Autodesk Inventor part; units mm, degrees
ref_plane "YZ Plane" through (0, 0, 0) normal (1, 0, 0) x (0, 1, 0)
ref_plane "XZ Plane" through (0, 0, 0) normal (0, 1, 0) x (-1, 0, 0)
ref_plane "XY Plane" through (0, 0, 0) normal (0, 0, 1) x (1, 0, 0)
sketch "スケッチ1" plane through (0, 0, 0) normal (0, 0, 1) x (1, 0, 0)
  circle A0 centre (0, 0) radius 18.4
extrude "押し出し1" add sketch "スケッチ1" along normal blind 24
sketch "スケッチ2" plane through (0, 0, 0) normal (0, 0, -1) x (-1, 0, 0)
  circle A0 centre (0, 0) radius 17.4
  dimension "d3" = 34.8
extrude "押し出し2" add sketch "スケッチ2" along normal blind 30.7
sketch "スケッチ3" plane through (0, 0, -30.7) normal (0, 0, -1) x (-1, 0, 0)
  circle A0 centre (0, 0) radius 17
  dimension "d6" = 34
extrude "押し出し3" add sketch "スケッチ3" along normal blind 15.4
sketch "スケッチ4" plane through (0, 0, 24) normal (0, 0, 1) x (1, 0, 0)
  circle A0 centre (0, -7) radius 6
  circle A1 centre (0, -7) radius 3
  point P0 (0, 0)
  point P1 (-15.5, 0)
  point P2 (0, 0)
  point P3 (-7.75, -13.4234)
  point P4 (7.75, -13.4234)
  point P5 (15.5, 0)
  point P6 (7.75, 13.4234)
  point P7 (-7.75, 13.4234)
  dimension "d11" = 360
  dimension "d13" = 15.5
  dimension "d14" = 7
  dimension "d15" = 12
  dimension "d16" = 6
extrude "押し出し4" add sketch "スケッチ4" along normal blind 6
extrude "押し出し5" add sketch "スケッチ4" along normal blind 22 contours A1
sketch "スケッチ5" plane through (0, -7, 46) normal (0, 0, 1) x (1, 0, 0)
  circle A0 centre (0, 0) radius 3
  line L0 (0, 2.4) -> (1.8, 2.4)
  line L1 (0, 2.4) -> (-1.8, 2.4)
  point P0 (0, 7)
  dimension "d21" = 6
  dimension "d22" = 2.4
extrude "押し出し6" cut sketch "スケッチ5" against normal blind 12 contours L0 L1 A0 picked at (-1.016, 2.5094)
sketch "スケッチ6" plane through (0, 0, 24) normal (0, 0, 1) x (1, 0, 0)
  point P0 (0, 0)
  point P1 (-15.5, 0)
  point P2 (-7.75, -13.4234)
  point P3 (7.75, -13.4234)
  point P4 (15.5, 0)
  point P5 (7.75, 13.4234)
  point P6 (-7.75, 13.4234)
  dimension "d25" = 15.5
  dimension "d28" = 360
hole "穴1" at (7.75, 13.4234, 24) at (-7.75, 13.4234, 24) at (-15.5, 0, 24) at (-7.75, -13.4234, 24) at (7.75, -13.4234, 24) at (15.5, 0, 24) direction (0, 0, -1) diameter 2.459 depth 8.8 tip angle 118
properties part number "Metal Gearmotor"
Read the model definition and answer for the solid it produces. Units are mm, in the model's axes. A direction names the side the tool comes from. Give positions to 0.01 mm unless a question says otherwise; leave off trailing zeros. Order: outer loops, then holes, each group sorted by start corner. A loop starts at its lowest first (then second) coordinate and runs counter-clockwise, first axis right, second up. Notation, with made-up numbers: (82.5, -28.5) -> (126.5, -28.5) arc R31 ccw to (126.5, -4.5) -> close; hole circle Ø8 at (41.5, 5.25). An arc over 180 degrees is marked (long way). One line per item, written item: value. Start each with the question number.
(1) The part is cut by section D-D (z = -17). Determine the outline of the cut face in (x, y).
(2) The part is cut by section C-C (y = -3). Determine the outline of the cut face in (x, z).
(3) A tool of negligible diameter and unlimited length cuts with its end or side. For faces 1 (the flat face through (0, -4.6, 40)), 2 (the cylindrical face through (-14.6, 11.2, 11.8)), 3 (the flat face through (0, 0, -46.1)), 4 (the cylindrical face through (8.5, 14.4, 19.5)), 5 (the flat face through (14, 11, 0)), from which of +Z, -Z, +X, -X, +Y, -Y can it reach the whole face along a straight path? Write none if from no direction.
(4) For a pull along X with two mould halves and no side action, classify faces 6 (the cylindrical face through (-6.55, 13.69, 19.54)), 7 (the cylindrical face through (-9.139, -14.334, -38.292)), 8 (the flat face through (-15.4, -7.7, -30.7)), 9 (the cylindrical face through (8.5, -12.45, 19.54)) as released by +X, released by -X, zero draft, split by the parting line, or undercut.
(5) The part is cut by section A-A (x = 0). Determine the outline of the cut face in (y, z), and give its area (3 significant figures).
(6) Flat-ended cylindrical pins translate along their axes: P1, Ø1, axis at y = 6.5, z = 11, coming from the -X side; P2, Ø12, axis at x = -9.5, z = 31, coming from the -Y side; P3, Ø2, axis at x = -7.75, y = -13.42, coming from the +Z side; P4, Ø6, axis at x = 1, y = -4.5, coming from the +Z side. Find the tip coordinate at first contact, or state that the pin passes through.
(7) Straight lines are drawn through the part: L1, parallel to Y at x = 7, z = 21; L2, parallel to X at y = -6, z = 16; L3, parallel to Y at x = -7.75, z = 20.75. For each, find the intervals that lie inside material, in ascending order.
(8) The part is cut by section B-B (z = -36.5). Determine the outline of the cut face in (x, y), and give its area (3 significant figures).
Taken from the geometry:
1. outline: circle Ø34.8 at (0, 0)
2. outline: (-18.15, 0) -> (-17.14, 0) -> (-17.14, -30.7) -> (-16.73, -30.7) -> (-16.73, -46.1) -> (16.73, -46.1) -> (16.73, -30.7) -> (17.14, -30.7) -> (17.14, 0) -> (18.15, 0) -> (18.15, 24) -> (4.47, 24) -> (4.47, 30) -> (-4.47, 30) -> (-4.47, 24) -> (-18.15, 24) -> close
3. face 1: +Z, +X, -X, +Y
3. face 2: +Z, -Z
3. face 3: -Z, +X, -X, +Y, -Y
3. face 4: +Z
3. face 5: -Z
4. face 6: undercut
4. face 7: split by the parting line
4. face 8: zero draft
4. face 9: undercut
5. outline: (-18.4, 0) -> (-17.4, 0) -> (-17.4, -30.7) -> (-17, -30.7) -> (-17, -46.1) -> (17, -46.1) -> (17, -30.7) -> (17.4, -30.7) -> (17.4, 0) -> (18.4, 0) -> (18.4, 24) -> (-1, 24) -> (-1, 30) -> (-4, 30) -> (-4, 34) -> (-4.6, 34) -> (-4.6, 46) -> (-10, 46) -> (-10, 30) -> (-13, 30) -> (-13, 24) -> (-18.4, 24) -> close
5. area: 2,640 mm^2
6. P1: x = -17.39
6. P2: y = -11.81
6. P3: z = 15.06
6. P4: z = 46
7. L1: -17.02 to -14.4, -12.45 to 12.45, 14.4 to 17.02
7. L2: -17.39 to 17.39
7. L3: -16.69 to -14.65, -12.19 to 12.19, 14.65 to 16.69
8. outline: circle Ø34 at (0, 0)
8. area: 908 mm^2
